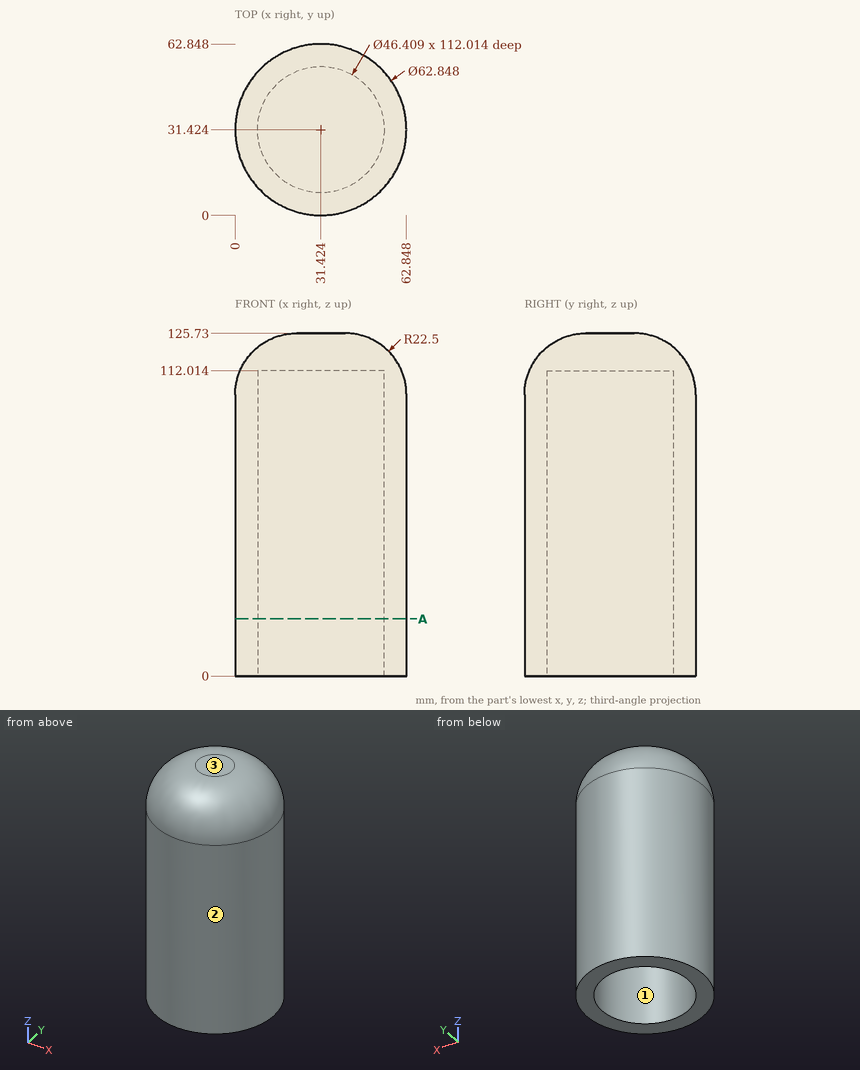
Check sheet for the drawn part. Datum: minimum x, y, z corner. Units: mm. Give positions to 0.01 mm unless a question says otherwise; leave off trailing zeros. Order: outer loops, then holes, each group sorted by start corner. A loop starts at its lowest first (then second) coordinate and runs counter-clockwise, first axis right, second up. Notation, with made-up numbers: (-8.5, -29) -> (18.5, -29) arc R33 ccw to (18.5, 4) -> close; hole circle Ø10 at (82, 11). An arc over 180 degrees is marked (long way). Use a Markdown table: item, result.
1) Mould release check, pull along Y, two halves, no side actions. Record for the marked faces 1, 2 and 3: pulls with the +Y half, pulls with the -Y half, needs draft (parallel to the pull), parting line crosses it, or undercut.
Results:
| item | result |
|---|---|
| face 1 | undercut |
| face 2 | parting line crosses it |
| face 3 | needs draft |
2) Depth check by flat-ended pin: pin 1 Ø10 at (x, y) = (31.5, 53) entering from +Z; pin 2 Ø3 at (x, y) = (38, 12.5) entering from -Z; pin 3 Ø2 at (x, y) = (12.5, 54) entering from +Z (1 decimal). Enter the tip coordinate at first touch or a pass-through.
Results:
| item | result |
|---|---|
| pin 1 | z = 124.39 |
| pin 2 | z = 112.01 |
| pin 3 | z = 114.4 |
3) Section check A-A, the plane z = 21. Record the boundary of the cut face in (x, y) (1 decimal), then the cut area to 3 significant figures.
Results:
| item | result |
|---|---|
| outline | circle Ø62.8 at (31.4, 31.4); hole circle Ø46.4 at (31.4, 31.4) |
| area | 1,410 mm² |
4) Material ranges on probe 1 along X at (y, z) = (24, 94.5); probe 2 along Y at (x, z) = (19, 35) (1 decimal); probe 3 along Y at (x, z) = (46, 67.5) (1 decimal), recorded low to high.
Results:
| item | result |
|---|---|
| probe 1 | 0.89 to 9.44, 53.41 to 61.96 |
| probe 2 | 2.6 to 11.8, 51 to 60.3 |
| probe 3 | 3.6 to 13.4, 49.5 to 59.3 |
